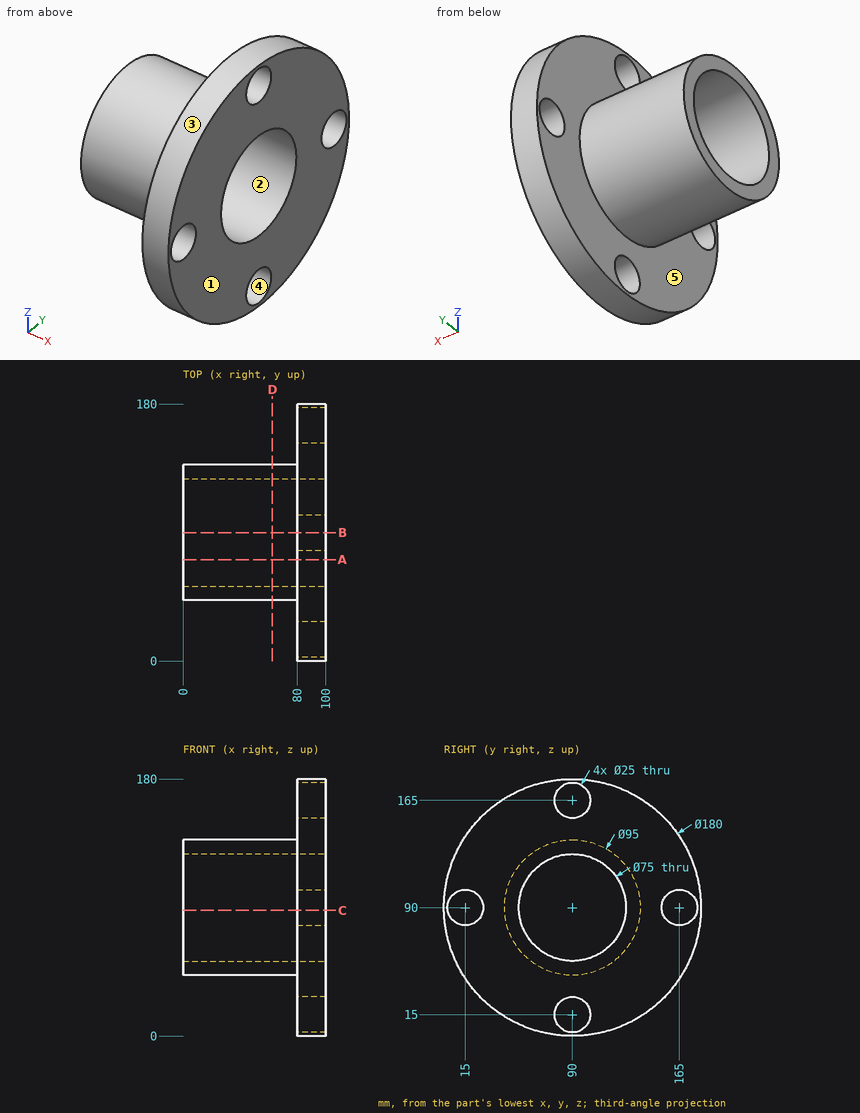
The figure shows three views and two pictorial views of one solid part (mm, origin at its lowest corner). Answer the questions. A direction names the side the tool comes from. Round coordinates to 2 decimals unless told otherwise and drop trailing zeros. Loops run counter-clockwise (first coordinate to the right, second up) from the corner with the lowest first, then second, coordinate; pieces in that order, holes last. Notation, with made-up numbers: M 53.5,41 L 104.5,41 A9 cw 104.5,53 Z; hole C 4,88 d9. An arc over 180 degrees is marked long. Use CSV: the item, a comma, the result in double quotes.
Q1. The mould has two halves that part along Y. Classify the marked faces 1, 2 and 3: pulls with the +Y half, pulls with the -Y half, needs draft (parallel to the pull), parting line crosses it, or undercut.
Determined:
face 1,"needs draft"
face 2,"undercut"
face 3,"parting line crosses it"
Q2. Section C-C, the plane z = 88 is taken. Determine the outline of the cut face in (x, y), then the cut area to 3 significant figures.
Determined:
outline,"M 0,42.54 L 80,42.54 L 80,27.34 L 100,27.34 L 100,52.55 L 0,52.55 Z; M 0,127.45 L 100,127.45 L 100,152.66 L 80,152.66 L 80,137.46 L 0,137.46 Z; M 80,0.02 L 100,0.02 L 100,2.66 L 80,2.66 Z; M 80,177.34 L 100,177.34 L 100,179.98 L 80,179.98 Z"
area,"2,720 mm2"
Q3. A tool of negligible diameter and unlimited length cuts with its end or side. For the marked faces 4 and 5, from which of +Z, -Z, +X, -X, +Y, -Y can it reach the whole face along a straight path? Write none if from no direction.
Determined:
face 4,"+X, -X"
face 5,"-X"
Q4. Section A-A, the plane y = 71 is taken. Determine the outline of the cut face in (x, z).
Determined:
outline,"M 0,46.47 L 80,46.47 L 80,2.03 L 100,2.03 L 100,57.67 L 0,57.67 Z; M 0,122.33 L 100,122.33 L 100,177.97 L 80,177.97 L 80,133.53 L 0,133.53 Z"
Q5. Section B-B, the plane y = 90 is taken. Determine the outline of the cut face in (x, z), then the cut area to 3 significant figures.
Determined:
outline,"M 0,42.5 L 80,42.5 L 80,27.5 L 100,27.5 L 100,52.5 L 0,52.5 Z; M 0,127.5 L 100,127.5 L 100,152.5 L 80,152.5 L 80,137.5 L 0,137.5 Z; M 80,0 L 100,0 L 100,2.5 L 80,2.5 Z; M 80,177.5 L 100,177.5 L 100,180 L 80,180 Z"
area,"2,700 mm2"
Q6. Consider L1, parallel to Y at x = 94, z = 90; L2, parallel to Y at x = 22.5, z = 90; L3, parallel to X at y = 125, z = 144.5. Determine where each line is inside the solid, lowest interval first.
Determined:
L1,"0 to 2.5, 27.5 to 52.5, 127.5 to 152.5, 177.5 to 180"
L2,"42.5 to 52.5, 127.5 to 137.5"
L3,"80 to 100"
Q7. Each of these flat-tipped pins is pushed along its axis until it touches: pin 1 (1 mm diameter, centred on x = 65.5, y = 114.5, fed in from +Z); pin 2 (6 mm diameter, centred on x = 74.5, y = 44.5, fed in from -Z); pin 3 (10 mm diameter, centred on y = 121.5, z = 150, fed in from -X). Where does it stop, or does it pass through?
Determined:
pin 1,"z = 130.99"
pin 2,"z = 68.79"
pin 3,"x = 80"
Q8. Section D-D, the plane x = 62.5 is taken. Determine the outline of the cut face in (y, z).
Determined:
outline,"C 90,90 d95; hole C 90,90 d75"
